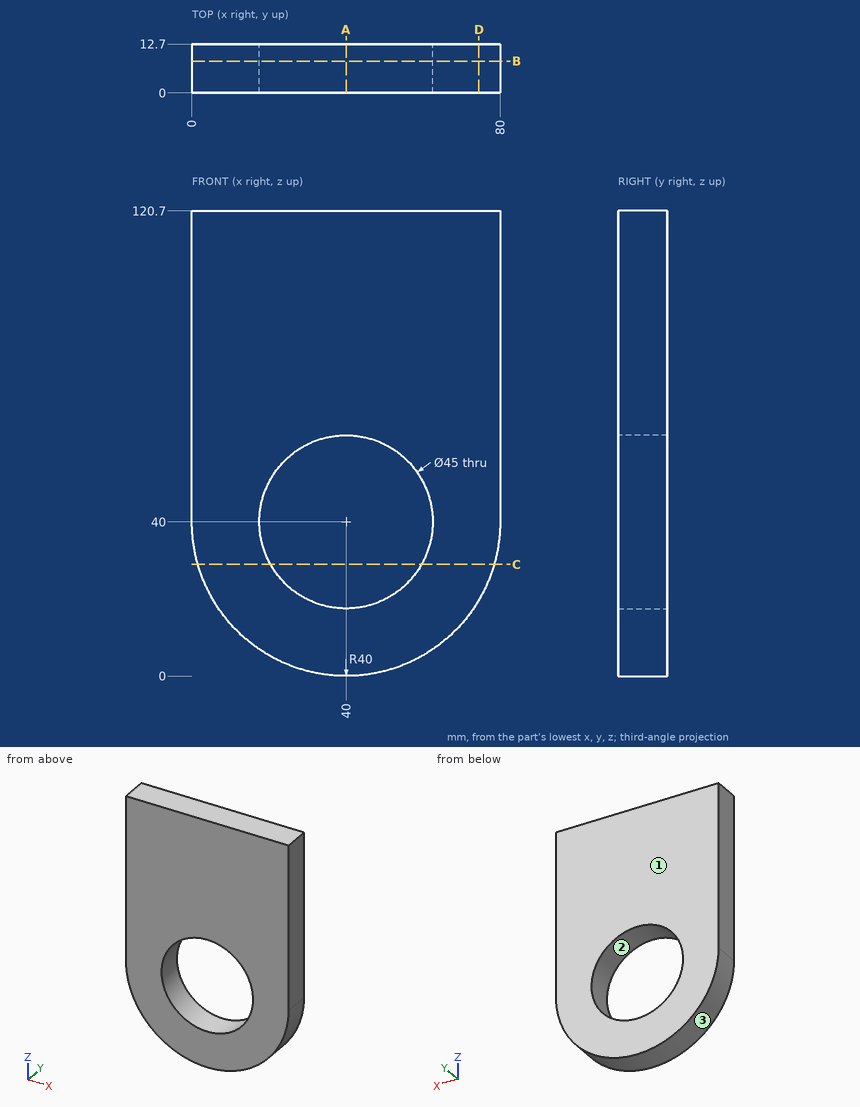
Geometry check sheet. Reference: drawing and pictorial views, mm from the part's lowest x, y, z. Give positions to 0.01 mm unless a question says otherwise; leave off trailing zeros. Loops run counter-clockwise (first coordinate to the right, second up) from the corner with the lowest first, then second, coordinate; pieces in that order, holes last. Notation, with made-up numbers: (53, 29.5) -> (90, 29.5) arc R29 cw to (90, 61.5) -> close; hole circle Ø1 at (11, 48.5). An arc over 180 degrees is marked (long way). Answer in a Markdown table with one row per item. Add a question column.
1) Cross-section at D-D on x = 74.5. Record the boundary of the cut face in (y, z).
2) Cross-section at B-B on y = 8.25. Record the boundary of the cut face in (x, z).
3) Draft check along X on the marked faces 1, 2 and 3. Enter one of: pulls with the +X half, pulls with the -X half, needs draft (parallel to the pull), parting line crosses it, or undercut.
4) Material ranges on probe 1 along X at (y, z) = (6, 40); probe 2 along Z at (x, y) = (33.5, 7.5); probe 3 along Z at (x, y) = (44, 7.5), recorded low to high. Write a range as from..to.
5) Gauge pin test, flat ends, axial feed: P1, Ø1.5, axis at x = 15.5, y = 11, coming from the -Z side; P2, Ø1.5, axis at x = 27, y = 10.5, coming from the -Z side. Record the tip position at first contact, or that the pin passes through.
6) Cross-section at C-C on z = 29. Record the boundary of the cut face in (x, y).
7) Cross-section at A-A on x = 40. Record the boundary of the cut face in (y, z).
Outcome:
| question | item | result |
|---|---|---|
| 1 | outline | (0, 19.76) -> (12.7, 19.76) -> (12.7, 120.7) -> (0, 120.7) -> close |
| 2 | outline | (0, 40) arc R40 ccw to (80, 40) -> (80, 120.7) -> (0, 120.7) -> close; hole circle Ø45 at (40, 40) |
| 3 | face 1 | needs draft |
| 3 | face 2 | undercut |
| 3 | face 3 | parting line crosses it |
| 4 | probe 1 | x = 0..17.5, 62.5..80 |
| 4 | probe 2 | z = 0.53..18.46, 61.54..120.7 |
| 4 | probe 3 | z = 0.2..17.86, 62.14..120.7 |
| 5 | P1 | stops at z = 7.81 |
| 5 | P2 | stops at z = 1.92 |
| 6 | outline | (1.54, 0) -> (20.37, 0) -> (20.37, 12.7) -> (1.54, 12.7) -> close; (59.63, 0) -> (78.46, 0) -> (78.46, 12.7) -> (59.63, 12.7) -> close |
| 7 | outline | (0, 0) -> (12.7, 0) -> (12.7, 17.5) -> (0, 17.5) -> close; (0, 62.5) -> (12.7, 62.5) -> (12.7, 120.7) -> (0, 120.7) -> close |
